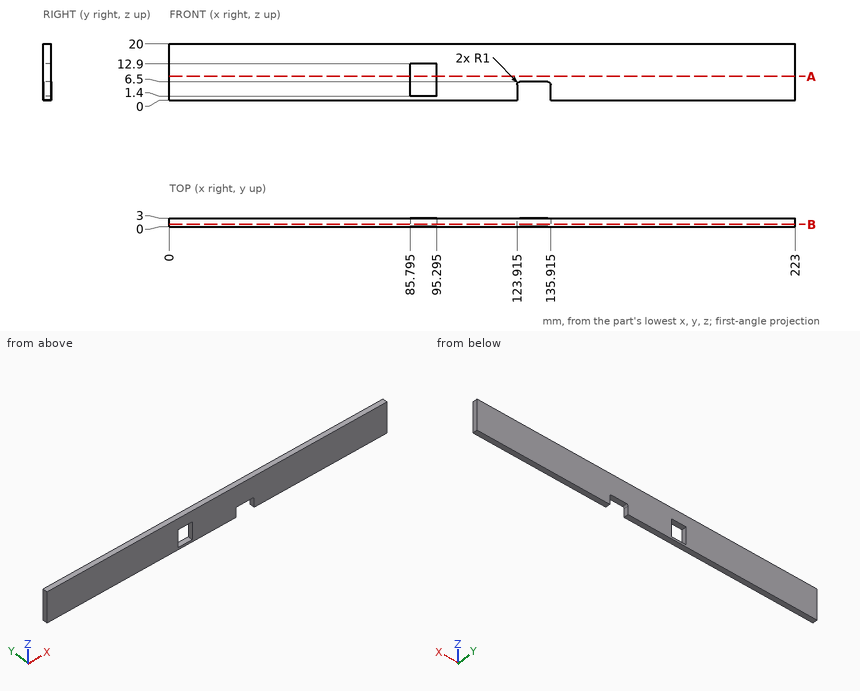
Could you check a few things on this drawing? It's one solid part, dimensions in mm from its lowest x, y, z. Give positions to 0.01 mm unless a question says otherwise; leave off trailing zeros. Loops run counter-clockwise (first coordinate to the right, second up) from the corner with the lowest first, then second, coordinate; pieces in that order, holes last. Notation, with made-up numbers: M 37.5,-36 L 86.5,-36 A14 ccw 86.5,-14 Z; hole C 72.25,54.5 d5. An arc over 180 degrees is marked long. One line per question, with ' | ' between items. Start each with the question number.
Q1. If we section it at A-A (z = 8.5): Please give me the cut outline in (x, y) (3 decimals).
Q2. If I drill on line 1 (X direction, y = 1.55, z = 5.75) (3 decimals); line 2 (X direction, y = 2.5, z = 7.5) (3 decimals); line 3 (X direction, y = 0.7, z = 6) (3 decimals), over which ranges is the centre line in solid material (lowest first)? Write a range as from..to.
Q3. If we section it at B-B (y = 0.75): Please give me the cut outline in (x, z) (3 decimals), plus the area to 3 significant figures.
Q4. For pin 1 Ø2 at (x, z) = (24.5, 12.5) entering from -Y, with a flat end and sliding along its axis, tell me the tip position at first contact or that it passes through.
Computed:
1) outline: M 0,0 L 85.795,0 L 85.795,3 L 0,3 Z; M 95.295,0 L 223,0 L 223,3 L 95.295,3 Z
2) line 1: x = 0..85.795, 95.295..123.947, 135.883..223 | line 2: x = 0..85.795, 95.295..223 | line 3: x = 0..85.795, 95.295..124.049, 135.781..223
3) outline: M 0,0 L 123.915,0 L 123.915,5.5 A1 cw 124.915,6.5 L 134.915,6.5 A1 cw 135.915,5.5 L 135.915,0 L 223,0 L 223,20 L 0,20 Z; hole M 85.795,1.4 L 95.295,1.4 L 95.295,12.9 L 85.795,12.9 Z | area: 4,270 mm²
4) pin 1: stops at y = 0
